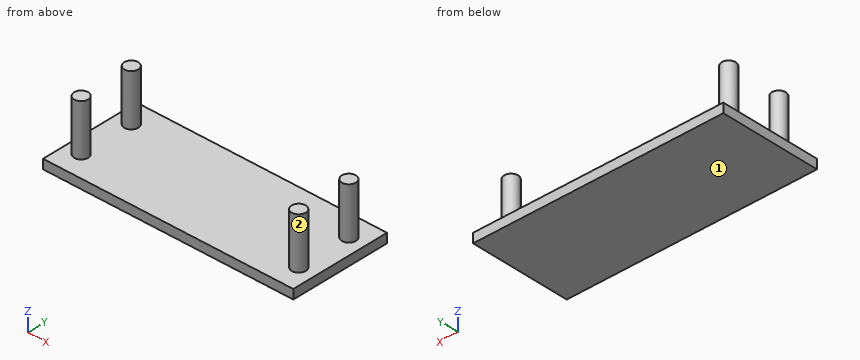
from build123d import *

# Parameters (mm, degrees)
F0_W     = 1358.9
F0_H     = 546.1
F1_DEPTH = 50.8
F2_R     = 38.1
F3_DEPTH = 330.2


with BuildPart() as f1:
    # F0 (on Top) → F1 (new body)
    with BuildSketch(Plane.XY):
        with Locations((679.45, 273.05)):
            Rectangle(F0_W, F0_H)
    extrude(amount=F1_DEPTH)

    # F2 (on face) → F3 (join)
    with BuildSketch(Plane(origin=(0, 0, 0), x_dir=(1, 0, 0), z_dir=(0, 0, -1))):
        with Locations((88.9, -127)):
            Circle(F2_R)
        with Locations((1270, -127)):
            Circle(F2_R)
        with Locations((88.9, -419.1)):
            Circle(F2_R)
        with Locations((1270, -419.1)):
            Circle(F2_R)
    extrude(amount=-F3_DEPTH)


solid = f1.part
Can you work these out from the model? Positions are in its coordinate system, mm. Face numbers are marked on the shaded views. Give positions to 0.01 mm unless a question says otherwise; leave off trailing zeros. Order: outer loops, then holes, each group sorted by start corner. A loop starts at its lowest first (then second) coordinate and runs counter-clockwise, first axis right, second up. Notation, with made-up numbers: M 67,78.25 L 71,78.25 A29 cw 71,114.25 Z; hole C 27,80.25 d4. An arc over 180 degrees is marked long. Use one line per item in the form item = value. Start each with the question number.
Item 1: If I drill on line 1 along Z through (x, y) = (567, 486.5); line 2 along X through (y, z) = (128.5, 136.5); line 3 along X through (y, z) = (155, 293), over which ranges is the centre line in solid material (lowest first)?
Item 2: If we section it at B-B (x = 88.9): Write out the boundary of the cut face in (y, z).
Item 3: If we section it at A-A (y = 127): Write out the boundary of the cut face in (x, z).
Item 4: If we section it at D-D (y = 250): Write out the boundary of the cut face in (x, z).
Item 5: If we section it at C-C (z = 262): Write out the boundary of the cut face in (x, y).
Item 6: Will these pins go through, and if not, where does the flat tip stop? pin 1 Ø2 at (y, z) = (144.5, 144) entering from -X; pin 2 Ø1.5 at (x, y) = (622, 140.5) entering from +Z; pin 3 Ø2 at (y, z) = (134, 193.5) entering from -X.
Item 7: We'd pull the mould along X, two halves only. Please class the marked faces 1 and 2: +X half, -X half, draft (parallel to the pull), parting line (faces both ways), or undercut.
Outcome:
q1.line_1 = 0 to 50.8
q1.line_2 = 50.83 to 126.97, 1231.93 to 1308.07
q1.line_3 = 63.06 to 114.74, 1244.16 to 1295.84
q2.outline = M 0,0 L 546.1,0 L 546.1,50.8 L 457.2,50.8 L 457.2,330.2 L 381,330.2 L 381,50.8 L 165.1,50.8 L 165.1,330.2 L 88.9,330.2 L 88.9,50.8 L 0,50.8 Z
q3.outline = M 0,0 L 1358.9,0 L 1358.9,50.8 L 1308.1,50.8 L 1308.1,330.2 L 1231.9,330.2 L 1231.9,50.8 L 127,50.8 L 127,330.2 L 50.8,330.2 L 50.8,50.8 L 0,50.8 Z
q4.outline = M 0,0 L 1358.9,0 L 1358.9,50.8 L 0,50.8 Z
q5.outline = C 88.9,127 d76.2; C 88.9,419.1 d76.2; C 1270,127 d76.2; C 1270,419.1 d76.2
q6.pin_1 = 54.56
q6.pin_2 = 50.8
q6.pin_3 = 51.28
q7.face_1 = draft
q7.face_2 = undercut
